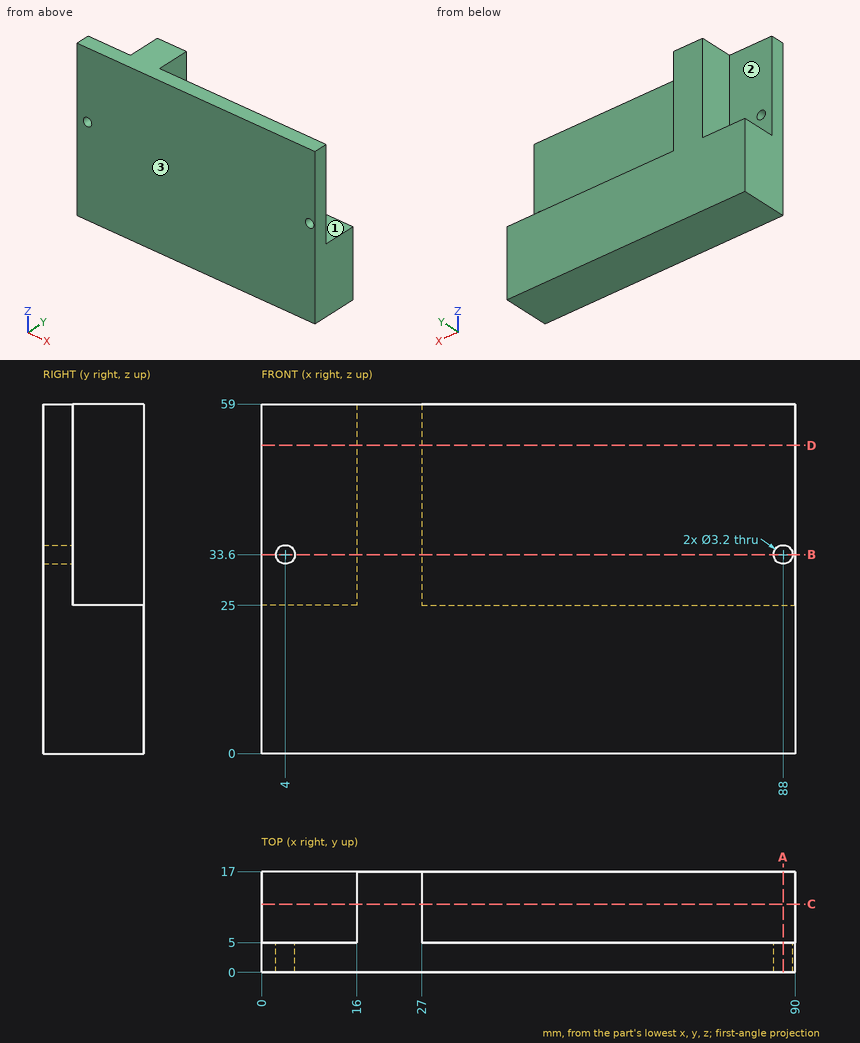
The figure shows three views and two pictorial views of one solid part (mm, origin at its lowest corner). Answer the questions. A direction names the side the tool comes from. Give positions to 0.01 mm unless a question says otherwise; leave off trailing zeros. Order: outer loops, then holes, each group sorted by start corner. A loop starts at its lowest first (then second) coordinate and runs counter-clockwise, first axis right, second up. Notation, with made-up numbers: (40, -22.5) -> (70, -22.5) arc R34 ccw to (70, 14.5) -> close; hole circle Ø11 at (-2.75, 26). An arc over 180 degrees is marked (long way). Answer as a JSON object with one key per item and string values. Group by question number.
Item 1: The part is cut by section D-D on z = 52. Write down the section's boundary in (x, y), and give its area (3 significant figures).
Item 2: Flat-ended cylindrical pins translate along their axes: pin 1 (10 mm diameter, centred on y = 14.5, z = 35.5, fed in from +X); pin 2 (5 mm diameter, centred on x = 11, z = 45, fed in from +Y); pin 3 (3.5 mm diameter, centred on y = 8.5, z = 34, fed in from -X). Find the tip coordinate at first contact, or state that the pin passes through.
Item 3: The part is cut by section A-A on x = 88. Write down the section's boundary in (y, z).
Item 4: The part is cut by section B-B on z = 33.6. Write down the section's boundary in (x, y).
Item 5: A tool of negligible diameter and unlimited length cuts with its end or side. For the marked faces 1, 2 and 3, from which of +Z, -Z, +X, -X, +Y, -Y can it reach the whole face along a straight path? Write none if from no direction.
Item 6: The part is cut by section C-C on y = 11.5. Write down the section's boundary in (x, z), and give its area (3 significant figures).
Item 7: Consider L1, parallel to X at y = 3.9, z = 33.6; L2, parallel to Z at x = 88, y = 3.4; L3, parallel to Y at x = 64, z = 49. Determine where each line is inside the solid, lowest interval first. Write a range as from..to.
Result set:
{
 "1": {"outline": "(0, 0) -> (90, 0) -> (90, 5) -> (27, 5) -> (27, 17) -> (16, 17) -> (16, 5) -> (0, 5) -> close", "area": "582 mm²"},
 "2": {"pin 1": "x = 27", "pin 2": "y = 5", "pin 3": "x = 16"},
 "3": {"outline": "(0, 0) -> (17, 0) -> (17, 25) -> (5, 25) -> (5, 32) -> (0, 32) -> close; (0, 35.2) -> (5, 35.2) -> (5, 59) -> (0, 59) -> close"},
 "4": {"outline": "(0, 0) -> (2.4, 0) -> (2.4, 5) -> (0, 5) -> close; (5.6, 0) -> (86.4, 0) -> (86.4, 5) -> (27, 5) -> (27, 17) -> (16, 17) -> (16, 5) -> (5.6, 5) -> close; (89.6, 0) -> (90, 0) -> (90, 5) -> (89.6, 5) -> close"},
 "5": {"face 1": "+Z, +X, +Y", "face 2": "+Z, -X, +Y", "face 3": "+Z, -Z, +X, -X, -Y"},
 "6": {"outline": "(0, 0) -> (90, 0) -> (90, 25) -> (27, 25) -> (27, 59) -> (16, 59) -> (16, 25) -> (0, 25) -> close", "area": "2,620 mm²"},
 "7": {"L1": "0..2.4, 5.6..86.4, 89.6..90", "L2": "0..32, 35.2..59", "L3": "0..5"}
}
